Model file for the job. Use its own axes, mm. Coordinates: 2 decimals unless noted, no trailing zeros. Write each loop counter-clockwise with the first axis right and the second up, starting at its lowest first coordinate (ties: lowest second). Pieces come first, ordered by that corner, then holes. Notation, with made-up numbers: (66.25, 80) -> (84.25, 80) arc R14 ccw to (84.25, 87) -> close; hole circle Ø11 at (8.25, 8). An arc over 180 degrees is marked (long way). Answer as a JSON object with one key per item and string values. Group by question number.
from build123d import *

# Parameters (mm, degrees)
F0_R     = 2.5
F0_R_2   = 4
F1_DEPTH = 5


with BuildPart() as f1:
    # F0 (on Front) → F1 (new body)
    with BuildSketch(Plane.XZ):
        Polygon((185.009293, 204.252433), (225.009293, 182.252433), (368.009293, 182.252433), (511.009293, 182.252433), (551.009293, 204.252433), (551.009293, 362.252433), (511.009293, 384.252433), (389.4801139832, 384.252433), (225.009293, 384.252433), (185.009293, 362.252433), align=None)
        with BuildLine():
            Line((211.509293, 251.752433), (217.509293, 251.752433))
            ThreePointArc((217.509293, 251.752433), (221.009293, 248.252433), (217.509293, 244.752433))
            Line((217.509293, 244.752433), (211.509293, 244.752433))
            ThreePointArc((211.509293, 244.752433), (208.009293, 248.252433), (211.509293, 251.752433))
        make_face(mode=Mode.SUBTRACT)
        with Locations((272.009293, 212.252433)):
            Circle(F0_R, mode=Mode.SUBTRACT)
        with BuildLine():
            ThreePointArc((270.5452164665, 338.0524329864), (278.8813852258, 351.8427530574), (294.060318, 357.252433))
            Line((294.060318, 357.252433), (388.009293, 357.252433))
            Line((388.009293, 357.252433), (441.958267, 357.252433))
            ThreePointArc((441.958267, 357.252433), (457.1371997667, 351.8427530635), (465.4733685296, 338.0524330052))
            ThreePointArc((465.4733685296, 338.0524330052), (469.9900217644, 306.8643277742), (470.8957123265, 275.3638866829))
            ThreePointArc((470.8957123265, 275.3638866829), (469.1970699877, 251.7911247549), (465.4733685296, 228.4524328857))
            ThreePointArc((465.4733685296, 228.4524328857), (457.1371997667, 214.6621128274), (441.958267, 209.2524328909))
            Line((441.958267, 209.2524328909), (368.0092925, 209.2524328909))
            Line((368.0092925, 209.2524328909), (294.060318, 209.2524328909))
            ThreePointArc((294.060318, 209.2524328909), (278.8813852287, 214.6621128311), (270.545216468, 228.4524328972))
            ThreePointArc((270.545216468, 228.4524328972), (265.7992173248, 262.4616912169), (265.3442938418, 296.797491833))
            ThreePointArc((265.3442938418, 296.797491833), (267.1610334487, 317.523764537), (270.5452164665, 338.0524329864))
        make_face(mode=Mode.SUBTRACT)
        with BuildLine():
            ThreePointArc((211.509293, 314.752433), (208.009293, 318.252433), (211.509293, 321.752433))
            Line((211.509293, 321.752433), (217.509293, 321.752433))
            ThreePointArc((217.509293, 321.752433), (221.009293, 318.252433), (217.509293, 314.752433))
            Line((217.509293, 314.752433), (211.509293, 314.752433))
        make_face(mode=Mode.SUBTRACT)
        with Locations((272.009293, 354.252433)):
            Circle(F0_R, mode=Mode.SUBTRACT)
        with Locations((368.009293, 363.252433)):
            Circle(F0_R_2, mode=Mode.SUBTRACT)
        with Locations((464.009293, 212.252433)):
            Circle(F0_R, mode=Mode.SUBTRACT)
        with BuildLine():
            Line((518.509293, 251.752433), (524.509293, 251.752433))
            ThreePointArc((524.509293, 251.752433), (528.009293, 248.252433), (524.509293, 244.752433))
            Line((524.509293, 244.752433), (518.509293, 244.752433))
            ThreePointArc((518.509293, 244.752433), (515.009293, 248.252433), (518.509293, 251.752433))
        make_face(mode=Mode.SUBTRACT)
        with Locations((477.009293, 283.252433)):
            Circle(F0_R_2, mode=Mode.SUBTRACT)
        with BuildLine():
            Line((524.509293, 314.752433), (518.509293, 314.752433))
            ThreePointArc((518.509293, 314.752433), (515.009293, 318.252433), (518.509293, 321.752433))
            Line((518.509293, 321.752433), (524.509293, 321.752433))
            ThreePointArc((524.509293, 321.752433), (528.009293, 318.252433), (524.509293, 314.752433))
        make_face(mode=Mode.SUBTRACT)
        with Locations((464.009293, 354.252433)):
            Circle(F0_R, mode=Mode.SUBTRACT)
    extrude(amount=F1_DEPTH)


solid = f1.part
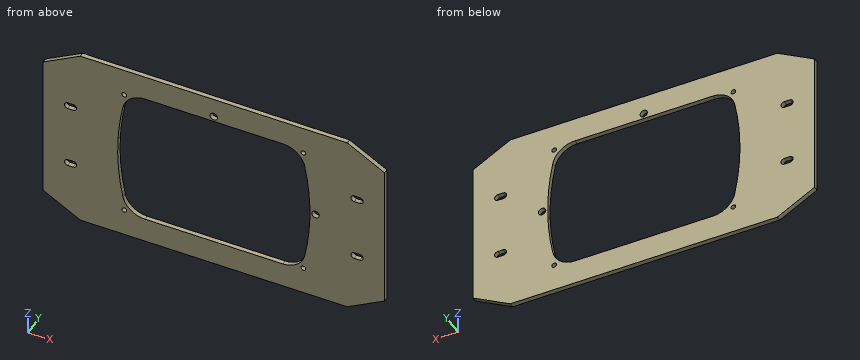
(1) Cut at B-B on z = 234.5. List the corners of the cut face in (x, y), plus the area to 3 significant figures.
(2) Cut at C-C on y = -1.55. Give the number of separate pieces and of enclosed holes in the cut face, plus the area to 3 significant figures.
(3) Pin check, flat tips, straight feed: pin 1 (2.5 mm diameter, centred on x = 522, y = -1.5, fed in from -Z); pin 2 (1.5 mm diameter, centred on x = 213, y = -1.5, fed in from -Z); pin 3 (1.5 mm diameter, centred on x = 522.5, y = -3.5, fed in from +Z). Stop position of each tip, or through.
(4) Cut at A-A on x = 384.5. List the corners of the cut face in (y, z).
(5) Wall check: probe 1 along Z at (x, y) = (355.5, -3.95); probe 2 along X at (y, z) = (-1.3, 319); probe 3 along X at (y, z) = (-3.5, 281.5). Give the ranges that are in metal, low to high.
Results found:
{
 "1": {"outline": "(185.01, -5) -> (269.38, -5) -> (269.38, 0) -> (185.01, 0) -> close; (466.64, -5) -> (551.01, -5) -> (551.01, 0) -> (466.64, 0) -> close", "area": "844 mm²"},
 "2": {"separate pieces": "1", "enclosed holes": "11", "area": "42,500 mm²"},
 "3": {"pin 1": "stops at z = 187.61", "pin 2": "stops at z = 188.45", "pin 3": "stops at z = 378.35"},
 "4": {"outline": "(-5, 182.25) -> (0, 182.25) -> (0, 209.25) -> (-5, 209.25) -> close; (-5, 357.25) -> (0, 357.25) -> (0, 384.25) -> (-5, 384.25) -> close"},
 "5": {"probe 1": "z = 182.25 to 209.25, 357.25 to 384.25", "probe 2": "x = 185.01 to 208.09, 220.93 to 267.35, 468.67 to 515.09, 527.93 to 551.01", "probe 3": "x = 185.01 to 265.01, 471 to 473.41, 480.6 to 551.01"}
}
